Read the model definition and answer for the solid it produces. Units are mm, in the model's axes. Face numbers are marked on the shaded views. A direction names the side the tool comes from. Give positions to 0.01 mm unless a question says otherwise; leave off trailing zeros. Order: outer loops, then holes, each group sorted by start corner. A loop starts at its lowest first (then second) coordinate and runs counter-clockwise, first axis right, second up. Notation, with made-up numbers: (35.25, 61.25) -> (78.25, 61.25) arc R29 cw to (78.25, 83.25) -> close; hole circle Ø11 at (-2.75, 5). An arc over 180 degrees is marked (long way). One line per item, written item: value. Start each with the question number.
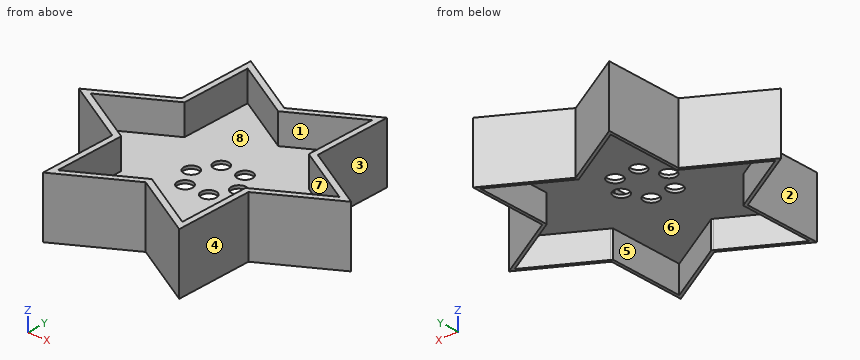
from build123d import *

# Parameters (mm, degrees)
F1_DEPTH     = 25.4
F2_T         = -2.54
F3_DEPTH     = 12.7
F4_T         = 1.27
F4_T3_DEPTH  = 27.94
F4_T5_DEPTH  = 33.2773657547
F4_T7_DEPTH  = 15.24
F4_T9_DEPTH  = 33.2773657547
F4_T11_DEPTH = 33.2773657547
F4_T13_DEPTH = 33.2773657547
F4_T15_DEPTH = 33.2773657547
F4_T17_DEPTH = 33.2773657547
F4_T19_DEPTH = 33.2773657547
F4_T21_DEPTH = 33.2773657547
F4_T23_DEPTH = 33.2773657547
F4_T25_DEPTH = 33.2773657547
F5_R         = 3.175
F6_DEPTH     = 25.4


# Not quite as in the source:
# - a shell that OpenCascade refuses in one call is made with other operations: the cavity is built on its own and cut out


with BuildPart() as f1:
    # F0 (on Top) → F1 (new body)
    with BuildSketch(Plane.XY):
        Polygon((-58.3186791779, 0), (-29.159339589, -16.8351525611), (-29.159339589, -50.5054576833), (0, -33.6703051222), (29.159339589, -50.5054576833), (29.159339589, -16.8351525611), (58.3186791779, 0), (29.159339589, 16.8351525611), (29.159339589, 50.5054576833), (0, 33.6703051222), (-29.159339589, 50.5054576833), (-29.159339589, 16.8351525611), align=None)
    extrude(amount=F1_DEPTH)

    # F2
    f2_openings = [f1.faces().sort_by_distance(p)[0] for p in [
        (0, 0, 25.4),
    ]]
    offset(amount=F2_T, openings=f2_openings, kind=Kind.INTERSECTION)

    # F0 (on Top) → F3 (join)
    with BuildSketch(Plane.XY):
        Polygon((-58.3186791779, 0), (-29.159339589, -16.8351525611), (-29.159339589, -50.5054576833), (0, -33.6703051222), (29.159339589, -50.5054576833), (29.159339589, -16.8351525611), (58.3186791779, 0), (29.159339589, 16.8351525611), (29.159339589, 50.5054576833), (0, 33.6703051222), (-29.159339589, 50.5054576833), (-29.159339589, 16.8351525611), align=None)
    extrude(amount=F3_DEPTH)

    # F4: shell of thickness 1.27, made by hand


with BuildPart() as f4_core1:
    # F4_t2: copy of F1
    add(f1.part)

    # the walls: a layer under each face that stays
    f4_faces = [f4_core1.faces().sort_by_distance(p)[0] for p in [
        (-43.7390093835, -8.4175762805, 12.7),
        (-29.159339589, -33.6703051222, 12.7),
        (-14.5796697945, -42.0878814027, 12.7),
        (14.5796697945, -42.0878814027, 12.7),
        (29.159339589, -33.6703051222, 12.7),
        (43.7390093835, -8.4175762805, 12.7),
        (43.7390093835, 8.4175762805, 12.7),
        (29.159339589, 33.6703051222, 12.7),
        (14.5796697945, 42.0878814027, 12.7),
        (-14.5796697945, 42.0878814027, 12.7),
        (-29.159339589, 33.6703051222, 12.7),
        (-54.4307672328, 0, 25.4),
        (-26.619339589, -30.7373657547, 19.05),
        (0, 0, 12.7),
        (-13.3096697945, -38.4217071934, 19.05),
        (13.3096697945, -38.4217071934, 19.05),
        (26.619339589, -30.7373657547, 19.05),
        (39.9290093835, -7.6843414387, 19.05),
        (39.9290093835, 7.6843414387, 19.05),
        (26.619339589, 30.7373657547, 19.05),
        (13.3096697945, 38.4217071934, 19.05),
        (-13.3096697945, 38.4217071934, 19.05),
        (-26.619339589, 30.7373657547, 19.05),
        (-39.9290093835, 7.6843414387, 19.05),
        (-39.9290093835, -7.6843414387, 19.05),
        (-43.7390093835, 8.4175762805, 12.7),
    ]]
    thicken(f4_faces, amount=-F4_T, mode=Mode.SUBTRACT)

    # F4_s4 → F4_t3 (cut)
    with BuildSketch(Plane.XY.offset(-1.27)):
        Polygon((-29.178389589, -16.8461510837), (-28.524339589, -15.7353002983), (-27.889339589, -16.1019177192), (-27.889339589, -16.8351525611), align=None)
        Polygon((0, -33.6923021674), (-0.635, -32.5704528594), (0, -32.2038354384), (0.635, -32.5704528594), align=None)
        Polygon((29.178389589, -16.8461510837), (27.889339589, -16.8351525611), (27.889339589, -16.1019177192), (28.524339589, -15.7353002983), align=None)
        Polygon((29.178389589, 16.8461510837), (28.524339589, 15.7353002983), (27.889339589, 16.1019177192), (27.889339589, 16.8351525611), align=None)
        Polygon((0, 33.6923021674), (0.635, 32.5704528594), (0, 32.2038354384), (-0.635, 32.5704528594), align=None)
        Polygon((-29.178389589, 16.8461510837), (-27.889339589, 16.8351525611), (-27.889339589, 16.1019177192), (-28.524339589, 15.7353002983), align=None)
    extrude(amount=F4_T3_DEPTH, mode=Mode.SUBTRACT)

    # F4_s6 → F4_t5 (cut)
    with BuildSketch(Plane.XZ.offset(14.0986828773)):
        Polygon((-26.606639589, 12.7127), (-27.889339589, 12.7), (-27.889339589, 11.43), (-26.619339589, 11.43), align=None)
        Polygon((26.606639589, 12.7127), (26.619339589, 11.43), (27.889339589, 11.43), (27.889339589, 12.7), align=None)
    extrude(amount=F4_T5_DEPTH, mode=Mode.SUBTRACT)

    # F4_s8 → F4_t7 (cut)
    with BuildSketch(Plane.XY.offset(11.43)):
        Polygon((-26.612989589, -46.0950501094), (-27.889339589, -46.106048632), (-27.889339589, -48.3057531576), (-25.984339589, -47.2059008948), align=None)
        Polygon((26.612989589, -46.0950501094), (25.984339589, -47.2059008948), (27.889339589, -48.3057531576), (27.889339589, -46.106048632), align=None)
        Polygon((53.2259791779, 0), (53.8736791779, -1.0998522628), (55.7786791779, 0), (53.8736791779, 1.0998522628), align=None)
        Polygon((26.612989589, 46.0950501094), (27.889339589, 46.106048632), (27.889339589, 48.3057531576), (25.984339589, 47.2059008948), align=None)
        Polygon((-26.612989589, 46.0950501094), (-25.984339589, 47.2059008948), (-27.889339589, 48.3057531576), (-27.889339589, 46.106048632), align=None)
        Polygon((-53.2259791779, 0), (-53.8736791779, 1.0998522628), (-55.7786791779, 0), (-53.8736791779, -1.0998522628), align=None)
    extrude(amount=F4_T7_DEPTH, mode=Mode.SUBTRACT)

    # F4_s10 → F4_t9 (cut)
    with BuildSketch(Plane(origin=(-12.2098175317, -7.0493414387, 0), x_dir=(0, 0, 1), z_dir=(-0.8660254038, -0.5, 0))):
        Polygon((12.7127, 26.606639589), (11.43, 26.619339589), (11.43, 27.889339589), (12.7, 27.889339589), align=None)
    extrude(amount=F4_T9_DEPTH, mode=Mode.SUBTRACT)

    # F4_s12 → F4_t11 (cut)
    with BuildSketch(Plane.XZ.offset(-47.376048632)):
        Polygon((-26.606639589, 12.7127), (-26.619339589, 11.43), (-27.889339589, 11.43), (-27.889339589, 12.7), align=None)
        Polygon((26.606639589, 12.7127), (26.619339589, 11.43), (27.889339589, 11.43), (27.889339589, 12.7), align=None)
    extrude(amount=F4_T11_DEPTH, mode=Mode.SUBTRACT)

    # F4_s14 → F4_t13 (cut)
    with BuildSketch(Plane(origin=(-12.2098175317, 7.0493414387, 0), x_dir=(0, 0, 1), z_dir=(-0.8660254038, 0.5, 0))):
        Polygon((12.7127, 26.606639589), (11.43, 26.619339589), (11.43, 27.889339589), (12.7, 27.889339589), align=None)
    extrude(amount=F4_T13_DEPTH, mode=Mode.SUBTRACT)

    # F4_s16 → F4_t15 (cut)
    with BuildSketch(Plane(origin=(41.0288616463, 23.688024316, 0), x_dir=(0, 0, 1), z_dir=(-0.8660254038, -0.5, 0))):
        Polygon((12.7127, 26.606639589), (11.43, 26.619339589), (11.43, 27.889339589), (12.7, 27.889339589), align=None)
    extrude(amount=F4_T15_DEPTH, mode=Mode.SUBTRACT)

    # F4_s18 → F4_t17 (cut)
    with BuildSketch(Plane(origin=(41.0288616463, -23.688024316, 0), x_dir=(0, 0, 1), z_dir=(-0.8660254038, 0.5, 0))):
        Polygon((12.7127, 26.606639589), (11.43, 26.619339589), (11.43, 27.889339589), (12.7, 27.889339589), align=None)
    extrude(amount=F4_T17_DEPTH, mode=Mode.SUBTRACT)

    # F4_s20 → F4_t19 (cut)
    with BuildSketch(Plane(origin=(12.2098175317, 7.0493414387, 0), x_dir=(0, 0, 1), z_dir=(0.8660254038, 0.5, 0))):
        Polygon((12.7127, 26.606639589), (11.43, 26.619339589), (11.43, 27.889339589), (12.7, 27.889339589), align=None)
    extrude(amount=F4_T19_DEPTH, mode=Mode.SUBTRACT)

    # F4_s22 → F4_t21 (cut)
    with BuildSketch(Plane(origin=(12.2098175317, -7.0493414387, 0), x_dir=(0, 0, 1), z_dir=(0.8660254038, -0.5, 0))):
        Polygon((12.7127, 26.606639589), (11.43, 26.619339589), (11.43, 27.889339589), (12.7, 27.889339589), align=None)
    extrude(amount=F4_T21_DEPTH, mode=Mode.SUBTRACT)

    # F4_s24 → F4_t23 (cut)
    with BuildSketch(Plane(origin=(-41.0288616463, -23.688024316, 0), x_dir=(0, 0, 1), z_dir=(0.8660254038, 0.5, 0))):
        Polygon((12.7127, 26.606639589), (11.43, 26.619339589), (11.43, 27.889339589), (12.7, 27.889339589), align=None)
    extrude(amount=F4_T23_DEPTH, mode=Mode.SUBTRACT)

    # F4_s26 → F4_t25 (cut)
    with BuildSketch(Plane(origin=(-41.0288616463, 23.688024316, 0), x_dir=(0, 0, 1), z_dir=(0.8660254038, -0.5, 0))):
        Polygon((12.7127, 26.606639589), (11.43, 26.619339589), (11.43, 27.889339589), (12.7, 27.889339589), align=None)
    extrude(amount=F4_T25_DEPTH, mode=Mode.SUBTRACT)


with BuildPart() as f1_1:
    add(f1.part)

    # what is left inside the walls is the cavity
    f4_cavity = [f4_core1.part.solids().sort_by_distance(p)[0] for p in [
        (13.94467, -8.050959, 11.4173),
    ]]
    add(f4_cavity, mode=Mode.SUBTRACT)

    # F5 (on face) → F6 (cut)
    with BuildSketch(Plane.XY.offset(12.7)):
        with Locations((5.08, 8.7988181024)):
            Circle(F5_R)
        with Locations((10.16, 0)):
            Circle(F5_R)
        with Locations((5.08, -8.7988181024)):
            Circle(F5_R)
        with Locations((-5.08, -8.7988181024)):
            Circle(F5_R)
        with Locations((-10.16, 0)):
            Circle(F5_R)
        with Locations((-5.08, 8.7988181024)):
            Circle(F5_R)
    extrude(amount=-F6_DEPTH, mode=Mode.SUBTRACT)


solid = f1_1.part
Item 1: Find the intervals of material crossed by line 1 (X direction, y = -19, z = 2.75); line 2 (X direction, y = 27, z = 16.5); line 3 (X direction, y = -35, z = 8.5), in increasing order. Write a range as from..to.
Item 2: Flat-ended cylindrical pins translate along their axes: pin 1 (1 mm diameter, centred on y = 37.5, z = 20, fed in from -X); pin 2 (14 mm diameter, centred on y = 30.5, z = 16.5, fed in from +X); pin 3 (1 mm diameter, centred on y = -16.5, z = 6.5, fed in from +X); pin 4 (6 mm diameter, centred on x = 30.5, z = 12.5, fed in from +Y). Find the tip coordinate at first contact, or state that the pin passes through.
Item 3: Find section B-B on y = -41.5. Write down the section's boundary in (x, z).
Item 4: For a pull along Z with two mould halves and no side action, classify the marked faces 6, 7 and 8 as +Z half, -Z half, draft (parallel to the pull), parting line (faces both ways), or undercut.
Item 5: Find section D-D on x = -5.08. Write down the section's boundary in (y, z).
Item 6: Find section A-A on z = 4.5. Write down the section's boundary in (x, y) (3 decimals).
Item 7: Find section C-C on y = -7. Write down the section's boundary in (x, z), then the cut area to 3 significant figures.
Item 8: A tool of negligible diameter and unlimited length cuts with its end or side. For the marked faces 1, 2, 3, 4 and 5, from which of +Z, -Z, +X, -X, +Y, -Y can it reach the whole face along a straight path? Write none if from no direction.
Checks:
1. line 1: -29.16..-27.89, 27.89..29.16
1. line 2: -29.16..-26.62, 26.62..29.16
1. line 3: -29.16..-27.89, -4.84..-2.3, 2.3..4.84, 27.89..29.16
2. pin 1: x = -29.16
2. pin 2: x = 29.16
2. pin 3: x = 30.61
2. pin 4: y = 50.51
3. outline: (-29.16, 0) -> (-27.89, 0) -> (-27.89, 11.43) -> (-16.1, 11.43) -> (-16.1, 0) -> (-13.56, 0) -> (-13.56, 25.4) -> (-18.64, 25.4) -> (-18.64, 12.7) -> (-26.62, 12.7) -> (-26.62, 25.4) -> (-29.16, 25.4) -> close; (13.56, 0) -> (16.1, 0) -> (16.1, 11.43) -> (27.89, 11.43) -> (27.89, 0) -> (29.16, 0) -> (29.16, 25.4) -> (26.62, 25.4) -> (26.62, 12.7) -> (18.64, 12.7) -> (18.64, 25.4) -> (13.56, 25.4) -> close
4. face 6: -Z half
4. face 7: draft
4. face 8: +Z half
5. outline: (-36.6, 0) -> (-35.14, 0) -> (-35.14, 11.43) -> (-11.97, 11.43) -> (-11.97, 12.7) -> (-33.67, 12.7) -> (-33.67, 25.4) -> (-36.6, 25.4) -> close; (-5.62, 11.43) -> (5.62, 11.43) -> (5.62, 12.7) -> (-5.62, 12.7) -> close; (11.97, 11.43) -> (35.14, 11.43) -> (35.14, 0) -> (36.6, 0) -> (36.6, 25.4) -> (33.67, 25.4) -> (33.67, 12.7) -> (11.97, 12.7) -> close
6. outline: (-58.319, 0) -> (-29.159, -16.835) -> (-29.159, -50.505) -> (0, -33.67) -> (29.159, -50.505) -> (29.159, -16.835) -> (58.319, 0) -> (29.159, 16.835) -> (29.159, 50.505) -> (0, 33.67) -> (-29.159, 50.505) -> (-29.159, 16.835) -> close; hole (-55.779, 0) -> (-27.889, -16.102) -> (-27.889, -48.306) -> (0, -32.204) -> (27.889, -48.306) -> (27.889, -16.102) -> (55.779, 0) -> (27.889, 16.102) -> (27.889, 48.306) -> (0, 32.204) -> (-27.889, 48.306) -> (-27.889, 16.102) -> close
7. outline: (-46.19, 0) -> (-43.65, 0) -> (-43.65, 11.43) -> (-7.7, 11.43) -> (-7.7, 12.7) -> (-41.11, 12.7) -> (-41.11, 25.4) -> (-46.19, 25.4) -> close; (-2.46, 11.43) -> (2.46, 11.43) -> (2.46, 12.7) -> (-2.46, 12.7) -> close; (7.7, 11.43) -> (43.65, 11.43) -> (43.65, 0) -> (46.19, 0) -> (46.19, 25.4) -> (41.11, 25.4) -> (41.11, 12.7) -> (7.7, 12.7) -> close
7. area: 291 mm2
8. face 1: +Z
8. face 2: +Z, -Z, -X, -Y
8. face 3: +Z, -Z, +X, +Y
8. face 4: +Z, -Z, +X, -Y
8. face 5: -Z
